Autodesk Inventor part; units mm, degrees
ref_plane "YZ Plane" through (0, 0, 0) normal (1, 0, 0) x (0, 1, 0)
ref_plane "XZ Plane" through (0, 0, 0) normal (0, 1, 0) x (-1, 0, 0)
ref_plane "XY Plane" through (0, 0, 0) normal (0, 0, 1) x (1, 0, 0)
sketch "Sketch1" plane through (0, 0, 0) normal (0, 0, 1) x (1, 0, 0)
  circle A0 centre (-76, 20.6153) radius 2
  circle A1 centre (76, 20.6157) radius 2
  line L0 (25.6401, -28.4) -> (25.6401, -22.3)
  line L1 (25.6401, -22.3) -> (24.1401, -22.3)
  line L2 (24.1401, -22.3) -> (24.1401, -19.1)
  line L3 (24.1401, -19.1) -> (31.1401, -19.1)
  line L4 (31.1401, -19.1) -> (31.1401, -22.3)
  line L5 (31.1401, -22.3) -> (29.6401, -22.3)
  line L6 (29.6401, -22.3) -> (29.6401, -28.4)
  line L7 (29.6401, -28.4) -> (40.1868, -28.4)
  line L8 (40.1868, -28.4) -> (40.1868, -31.6)
  line L9 (40.1868, -31.6) -> (70.1868, -31.6)
  line L10 (70.1868, -31.6) -> (70.1868, -28.4)
  line L11 (70.1868, -28.4) -> (85, -28.4)
  line L12 (85, -28.4) -> (85, 31.6)
  line L13 (85, 31.6) -> (70.6157, 31.6)
  arc A2 (56.2026, 31.6) -> (70.6157, 31.6) centre (63.4091, 28.6157) ccw
  line L14 (56.2026, 31.6) -> (33.0157, 31.6)
  arc A3 (18.603, 31.6) -> (33.0157, 31.6) centre (25.8094, 28.6153) ccw
  line L15 (18.603, 31.6) -> (-2.4569, 31.6)
  arc A4 (-16.8696, 31.6) -> (-2.4569, 31.6) centre (-9.6632, 28.6153) ccw
  line L16 (-16.8696, 31.6) -> (-38.2294, 31.6)
  arc A5 (-52.6422, 31.6) -> (-38.2294, 31.6) centre (-45.4358, 28.6153) ccw
  line L17 (-52.6422, 31.6) -> (-85, 31.6)
  line L18 (-85, 31.6) -> (-85, -28.4)
  line L19 (-85, -28.4) -> (-70, -28.4)
  line L20 (-70, -28.4) -> (-70, -31.6)
  line L21 (-70, -31.6) -> (-40, -31.6)
  line L22 (-40, -31.6) -> (-40, -28.4)
  line L23 (-40, -28.4) -> (-29.4533, -28.4)
  line L24 (-29.4533, -28.4) -> (-29.4533, -22.3)
  line L25 (-29.4533, -22.3) -> (-30.9533, -22.3)
  line L26 (-30.9533, -22.3) -> (-30.9533, -19.1)
  line L27 (-30.9533, -19.1) -> (-23.9533, -19.1)
  line L28 (-23.9533, -19.1) -> (-23.9533, -22.3)
  line L29 (-23.9533, -22.3) -> (-25.4533, -22.3)
  line L30 (-25.4533, -22.3) -> (-25.4533, -28.4)
  line L31 (-25.4533, -28.4) -> (-14.9066, -28.4)
  line L32 (-14.9066, -28.4) -> (-14.9066, -31.6)
  line L33 (-14.9066, -31.6) -> (15.0934, -31.6)
  line L34 (15.0934, -31.6) -> (15.0934, -28.4)
  line L35 (15.0934, -28.4) -> (25.6401, -28.4)
  circle A6 centre (-45.4358, 28.6153) radius 7.8
  circle A7 centre (-20.4358, 28.6153) radius 7.8
  circle A8 centre (4.5642, 28.6153) radius 7.8
  circle A9 centre (29.5642, 28.6153) radius 7.8
  line L36 (85, -28.4) -> (85, 41.6)
  line L37 (85, 41.6) -> (-85, 41.6)
  line L38 (-85, 41.6) -> (-85, -28.4)
  line L39 (-85, -28.4) -> (-70, -28.4)
  line L40 (-70, -28.4) -> (-70, -31.6)
  line L41 (-70, -31.6) -> (-40, -31.6)
  line L42 (-40, -31.6) -> (-40, -28.4)
  line L43 (-40, -28.4) -> (-29.4533, -28.4)
  line L44 (-29.4533, -28.4) -> (-29.4533, -22.3)
  line L45 (-29.4533, -22.3) -> (-30.9533, -22.3)
  line L46 (-30.9533, -22.3) -> (-30.9533, -19.1)
  line L47 (-30.9533, -19.1) -> (-23.9533, -19.1)
  line L48 (-23.9533, -19.1) -> (-23.9533, -22.3)
  line L49 (-23.9533, -22.3) -> (-25.4533, -22.3)
  line L50 (-25.4533, -22.3) -> (-25.4533, -28.4)
  line L51 (-25.4533, -28.4) -> (-14.9066, -28.4)
  line L52 (-14.9066, -28.4) -> (-14.9066, -31.6)
  line L53 (-14.9066, -31.6) -> (15.0934, -31.6)
  line L54 (15.0934, -31.6) -> (15.0934, -28.4)
  line L55 (15.0934, -28.4) -> (25.6401, -28.4)
  line L56 (25.6401, -28.4) -> (25.6401, -22.3)
  line L57 (25.6401, -22.3) -> (24.1401, -22.3)
  line L58 (24.1401, -22.3) -> (24.1401, -19.1)
  line L59 (24.1401, -19.1) -> (31.1401, -19.1)
  line L60 (31.1401, -19.1) -> (31.1401, -22.3)
  line L61 (31.1401, -22.3) -> (29.6401, -22.3)
  line L62 (29.6401, -22.3) -> (29.6401, -28.4)
  line L63 (29.6401, -28.4) -> (40.1868, -28.4)
  line L64 (40.1868, -28.4) -> (40.1868, -31.6)
  line L65 (40.1868, -31.6) -> (70.1868, -31.6)
  line L66 (70.1868, -31.6) -> (70.1868, -28.4)
  line L67 (85, -28.4) -> (70.1868, -28.4)
  circle A10 centre (76, 20.6157) radius 2
  circle A11 centre (-76, 20.6153) radius 2
  point P0 (0, 0)
  dimension "d0" = 25
  dimension "d1" = 25
  dimension "d2" = 25
  dimension "d3" = 70
extrude "Extrusion1" add sketch "Sketch1" along normal blind 6.2 contours L35 L34 L33 L32 L31 L30 L29 L28 L27 L26 L25 L24 L23 L22 L21 L20 L19 L18 L17 A5 L16 A7 A4 A8 L15 A3 A9 L14 A2 L13 L12 L11 L10 L9 L8 L7 L6 L5 L4 L3 L2 L1 L0 | L13 A2 L14 A9 A3 L15 A8 A4 A7 L16 A6 L17 L38 L37 L36
properties part number "caja_2_Lateral"
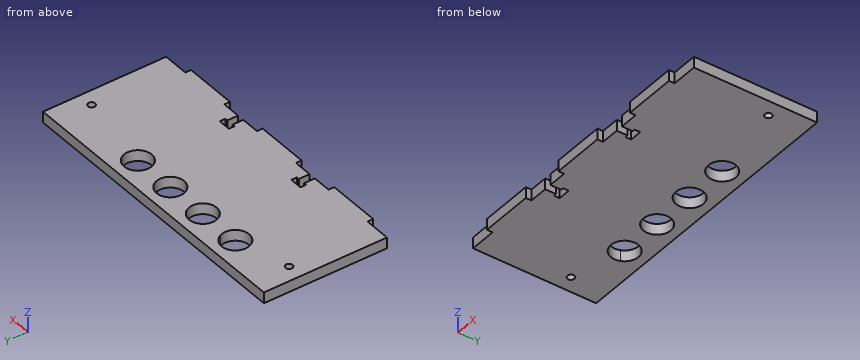
CAD build for the part. Positions are in the model's coordinates, mm. Coordinates: 2 decimals unless noted, no trailing zeros. Order: outer loops, then holes, each group sorted by start corner. A loop starts at its lowest first (then second) coordinate and runs counter-clockwise, first axis right, second up.
(1) Pin check, flat tips, straight feed: pin 1 Ø14 at (x, y) = (-20.44, 28.62) entering from -Z; pin 2 Ø3 at (x, z) = (-28.5, 4) entering from -Y; pin 3 Ø1 at (y, z) = (-30, 1.5) entering from -X; pin 4 Ø1 at (y, z) = (-30, 4.5) entering from +X. Stop position of each tip, or through.
Solution:
pin 1: passes through
pin 2: stops at y = -28.4
pin 3: stops at x = -70
pin 4: stops at x = 70.19
(2) Saw through at C-C, the plane x = -49. Write the cut outline in (y, z).
Solution:
outline: (-31.6, 0) - (21.68, 0) - (21.68, 6.2) - (-31.6, 6.2) - close; (35.55, 0) - (41.6, 0) - (41.6, 6.2) - (35.55, 6.2) - close
(3) Saw through at D-D, the plane z = 5. Count the separate pieces of the cut face and the enclosed holes in it, and give its area (3 significant figures).
Solution:
separate pieces: 1
enclosed holes: 6
area: 11,300 mm2
(4) Drill centre lines: L1, parallel to Y at x = 30, z = 5; L2, parallel to Y at x = 76, z = 2.75; L3, parallel to X at y = 34, z = 5. Where is each one in solid material? Low to high.
Solution:
L1: y = -28.4 to -22.3, -19.1 to 20.83, 36.4 to 41.6
L2: y = -28.4 to 18.62, 22.62 to 41.6
L3: x = -85 to -51.08, -39.79 to -26.08, -14.79 to -1.08, 10.21 to 23.92, 35.21 to 85
(5) Saw through at A-A, the plane x = -76. Write the cut outline in (y, z).
Solution:
outline: (-28.4, 0) - (18.62, 0) - (18.62, 6.2) - (-28.4, 6.2) - close; (22.62, 0) - (41.6, 0) - (41.6, 6.2) - (22.62, 6.2) - close
(6) Saw through at B-B, the plane y = 26.5. Write the cut outline in (x, z), and give its area (3 significant figures).
Solution:
outline: (-85, 0) - (-52.94, 0) - (-52.94, 6.2) - (-85, 6.2) - close; (-37.93, 0) - (-27.94, 0) - (-27.94, 6.2) - (-37.93, 6.2) - close; (-12.93, 0) - (-2.94, 0) - (-2.94, 6.2) - (-12.93, 6.2) - close; (12.07, 0) - (22.06, 0) - (22.06, 6.2) - (12.07, 6.2) - close; (37.07, 0) - (85, 0) - (85, 6.2) - (37.07, 6.2) - close
area: 682 mm2
